Geometry check sheet. Reference: drawing and pictorial views, mm from the part's lowest x, y, z. A direction names the side the tool comes from. Round coordinates to 2 decimals unless told otherwise and drop trailing zeros. Order: outer loops, then holes, each group sorted by start corner. A loop starts at its lowest first (then second) coordinate and runs counter-clockwise, first axis right, second up.
(1) Set-up check for the marked faces 5 and 6: record each of +Z, -Z, +X, -X, +Y, -Y from which the full face is reachable in a straight line by a thin tool's end or side.
(2) Sectioned sample at D-D (y = 26). Record the boundary of the cut face in (x, z) (1 decimal).
(3) Go/stop test with flat-tipped pins: pin 1 (4 mm diameter, centred on x = 11.075, z = 4.76, fed in from +Y); pin 2 (6 mm diameter, centred on x = 72.5, y = 9, fed in from +Z). Record where each tip stops, or that it passes through.
(4) Release check for a two-part mould opening along X. For the marked faces 1, 2, 3 and 4 record: +X half, -X half, draft (parallel to the pull), parting line (faces both ways), or undercut.
(5) Sectioned sample at A-A (x = 67). Record the boundary of the cut face in (y, z) (1 decimal), plus the area to 3 significant figures.
(6) Sectioned sample at B-B (y = 15.5). Record the boundary of the cut face in (x, z) (1 decimal).
(7) Material ranges on line 1 along X through (y, z) = (2.95, 4.76) (1 decimal); line 2 along Y through (x, z) = (75, 0.5); line 3 along X through (y, z) = (19, 6.25) (1 decimal), recorded low to high.
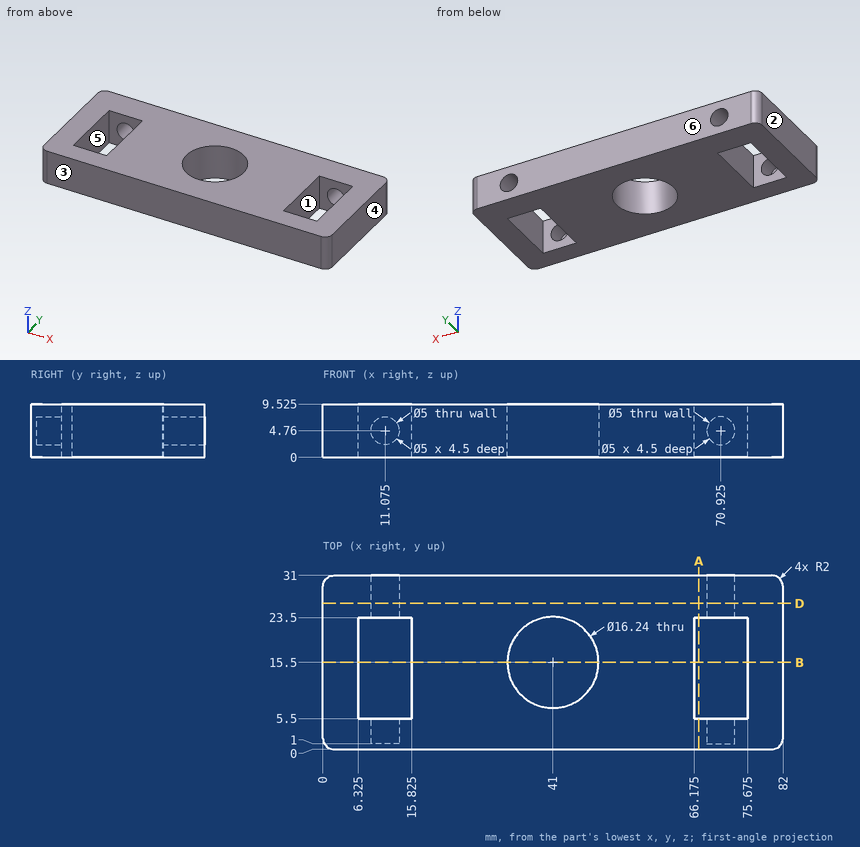
Answer below:
1. face 5: +Z, -Z
1. face 6: +Z, -Z, +X, -X, +Y
2. outline: (0, 0) - (82, 0) - (82, 9.5) - (0, 9.5) - close; hole circle Ø5 at (11.1, 4.8); hole circle Ø5 at (70.9, 4.8)
3. pin 1: stops at y = 1
3. pin 2: passes through
4. face 1: undercut
4. face 2: -X half
4. face 3: draft
4. face 4: +X half
5. outline: (0, 0) - (5.5, 0) - (5.5, 9.5) - (0, 9.5) - close; (23.5, 0) - (31, 0) - (31, 9.5) - (23.5, 9.5) - close
5. area: 124 mm2
6. outline: (0, 0) - (6.3, 0) - (6.3, 9.5) - (0, 9.5) - close; (15.8, 0) - (32.9, 0) - (32.9, 9.5) - (15.8, 9.5) - close; (49.1, 0) - (66.2, 0) - (66.2, 9.5) - (49.1, 9.5) - close; (75.7, 0) - (82, 0) - (82, 9.5) - (75.7, 9.5) - close
7. line 1: x = 0 to 8.6, 13.6 to 68.4, 73.4 to 82
7. line 2: y = 0 to 5.5, 23.5 to 31
7. line 3: x = 0 to 6.3, 15.8 to 33.7, 48.3 to 66.2, 75.7 to 82
